Design review of the part built by this model. Coordinates are the model's own, in mm. Round coordinates to 2 decimals unless told otherwise and drop trailing zeros. Loops run counter-clockwise (first coordinate to the right, second up) from the corner with the lowest first, then second, coordinate; pieces in that order, holes last. Notation, with made-up numbers: (80.25, 77.5) - (111.25, 77.5) arc R29 cw to (111.25, 112.5) - close; hole circle Ø11 at (2, 62.25). An arc over 180 degrees is marked (long way). Use one line per item in the form item = value. Start each with the question number.
(1) We need section C-C, the plane x = -13. Write out the cut boundary in (y, z), then the cut area to 3 significant figures.
(2) Wall thickness on probe 1 along X at (y, z) = (4.5, 2.4); probe 2 along X at (y, z) = (6, 1.45); probe 3 along X at (y, z) = (27, 1.25): over which ranges is each line inside the solid? List them lowest first. Write a range as [from, to].
(3) We need section D-D, the plane z = 1.7. Write out the cut boundary in (x, y).
(4) The part is to be moulded in two halves that separate along X. For faces 1 (the cylindrical face through (-0.617, 32.494, 1.479)), 2 (the cylindrical face through (25.71, 7.45, 1.48)), 3 (the flat face through (-3, 25, 0)), say which applies: released by +X, released by -X, zero draft, split by the parting line, or undercut.
(5) We need section A-A, the plane y = 12.5. Write out the cut boundary in (x, z).
(6) We need section B-B, the plane y = 26.5. Write out the cut boundary in (x, z), then the cut area to 3 significant figures.
(7) For pin 1 (1 mm diameter, centred on y = 10, z = 1.5, fed in from +X); pin 2 (1.5 mm diameter, centred on y = 13.5, z = 2.5, fed in from +X), all flat-tipped, find the tip position at first contact; note any pin that passes through.
Autodesk Inventor part; units mm, degrees
ref_plane "YZ Plane" through (0, 0, 0) normal (1, 0, 0) x (0, 1, 0)
ref_plane "XZ Plane" through (0, 0, 0) normal (0, 1, 0) x (-1, 0, 0)
ref_plane "XY Plane" through (0, 0, 0) normal (0, 0, 1) x (1, 0, 0)
sketch "Sketch1" plane through (0, 0, 0) normal (0, 0, 1) x (1, 0, 0)
  circle A0 centre (27.2972, 6.234) radius 2
  circle A1 centre (12.1456, 25.2286) radius 2
  circle A2 centre (-12.1519, 25.2256) radius 2
  circle A3 centre (-27.2988, 6.2272) radius 2
  circle A4 centre (-21.8891, -17.4604) radius 2
  circle A5 centre (0.0035, -28) radius 2
  circle A6 centre (21.8935, -17.455) radius 2
  arc A7 (-18.3712, -14.6543) -> (-25.407, -20.2666) centre (-21.8891, -17.4604) ccw
  arc A8 (-31.6861, 7.228) -> (-22.9115, 5.2264) centre (-27.2988, 6.2272) ccw
  line L0 (0, 0) -> (-27.2988, 6.2272)
  line L1 (0, 0) -> (-28.0096, 0)
  arc A9 (22.9102, 5.2321) -> (31.6843, 7.2359) centre (27.2972, 6.234) ccw
  arc A10 (25.412, -20.2603) -> (18.3749, -14.6497) centre (21.8935, -17.455) ccw
  arc A11 (18.3162, -14.7229) -> (18.3749, -14.6497) centre (0, 0) ccw
  arc A12 (22.9102, 5.2321) -> (-22.9115, 5.2264) centre (0, 0) ccw
  arc A13 (25.3999, -20.2755) -> (25.412, -20.2603) centre (0, 0) ccw
  arc A14 (31.6843, 7.2359) -> (-31.6861, 7.228) centre (0, 0) ccw
  arc A15 (31.3012, -23.1554) -> (15.9051, -8.2279) centre (21.8935, -17.455) ccw
  line L2 (21.8935, -17.455) -> (20.255, -16.308)
  line L3 (18.0457, -14.7615) -> (15.8179, -13.202)
  line L4 (21.8935, -17.455) -> (23.0905, -19.0572)
  line L5 (25.3705, -22.1091) -> (26.3321, -23.3962)
  arc A16 (25.3999, -20.2755) -> (25.3705, -22.1091) centre (26.5722, -21.2113) ccw
  arc A17 (26.3321, -23.3962) -> (31.3012, -23.1554) centre (28.7355, -21.6007) ccw
  arc A18 (15.9051, -8.2279) -> (15.8179, -13.202) centre (17.5383, -10.7444) ccw
  arc A19 (18.0457, -14.7615) -> (18.3162, -14.7229) centre (18.1604, -14.5976) ccw
  point P0 (28.477, -26.2673)
  point P1 (12.8819, -11.1468)
  point P2 (18.1984, -14.8684)
  point P3 (24.6644, -21.164)
  dimension "d2" = 4
  dimension "d5" = 360
  dimension "d7" = 9
  dimension "d8" = 9
  dimension "d11" = 12.85
  dimension "d12" = 54.596
  dimension "d13" = 9
  dimension "d14" = 22
  dimension "d15" = 1.5
  dimension "d16" = 3
  dimension "d17" = 0.2
extrude "Extrusion1" add sketch "Sketch1" along normal blind 3 contours A14 A9 A12 A8
properties part number "fin entraineur mod"
Data:
q1.outline = (19.58, 0) - (23.41, 0) - (23.41, 3) - (19.58, 3) - close; (27.04, 0) - (29.79, 0) - (29.79, 3) - (27.04, 3) - close
q1.area = 19.8 mm^2
q2.probe_1 = [-31.45, -28.31], [-26.29, -23.14], [23.14, 26.3], [28.29, 31.45]
q2.probe_2 = [-31.79, -29.29], [-25.31, -22.72], [22.72, 25.31], [29.28, 31.79]
q2.probe_3 = [-18.09, -13.07], [-11.23, 11.22], [13.07, 18.09]
q3.outline = (-31.69, 7.23) arc R4.5 ccw to (-22.91, 5.23) arc R23.5 cw to (22.91, 5.23) arc R4.5 ccw to (31.68, 7.24) arc R32.5 ccw to start; hole circle Ø4 at (-27.3, 6.23); hole circle Ø4 at (-12.15, 25.23); hole circle Ø4 at (12.15, 25.23); hole circle Ø4 at (27.3, 6.23)
q4.face_1 = split by the parting line
q4.face_2 = undercut
q4.face_3 = zero draft
q5.outline = (-30, 0) - (-19.9, 0) - (-19.9, 3) - (-30, 3) - close; (19.9, 0) - (30, 0) - (30, 3) - (19.9, 3) - close
q6.outline = (-18.81, 0) - (-13.69, 0) - (-13.69, 3) - (-18.81, 3) - close; (-10.61, 0) - (10.6, 0) - (10.6, 3) - (-10.61, 3) - close; (13.69, 0) - (18.81, 0) - (18.81, 3) - (13.69, 3) - close
q6.area = 94.4 mm^2
q7.pin_1 = 31.08
q7.pin_2 = 29.89
